```python
from build123d import *


with BuildPart() as part:
    # Sweep1: sweep along a path in Sketch1
    with BuildLine(Plane(origin=(0, 0, 0), x_dir=(1, 0, 0), z_dir=(0, 1, 0))) as sweep1_path:
        Line((0, 0), (25.4, 0))
        ThreePointArc((25.4, 0), (30.4, 1.339745962), (34.060254038, 5))
    # Sketch2 → Sweep1 (sweep)
    with BuildSketch(Plane(origin=(0, 0, 0), x_dir=(0, 0, -1), z_dir=(1, 0, 0))):
        with BuildLine():
            Line((0, 5), (0, -5))
            Line((0, -5), (-5, -5))
            ThreePointArc((-5, -5), (-3.974330816, 0), (-5, 5))
            Line((-5, 5), (0, 5))
        make_face()
    sweep(path=sweep1_path.line)


solid = part.part
```
The model under review builds one solid part; all positions refer to its coordinate system, in mm. A direction names the side the tool comes from. Round coordinates to 2 decimals unless told otherwise and drop trailing zeros. Loops run counter-clockwise (first coordinate to the right, second up) from the corner with the lowest first, then second, coordinate; pieces in that order, holes last.
1) Tool access review of faces 4 (the face through (13, 0, 0)), 5 (the face through (0, 0, 2)): name each direction out of +Z, -Z, +X, -X, +Y, -Y from which nothing blocks a thin tool from reaching the whole face with its end or side.
Values follow:
face 4: -Z, -X, +Y, -Y
face 5: +Z, -Z, -X, +Y, -Y
2) Wall thickness on line 1 along Z through (x, y) = (6.5, -3); line 2 along Z through (x, y) = (3, 0.25); line 3 along X through (y, z) = (4.75, -3.25): over which ranges is each line inside the solid? List them lowest first.
Values follow:
line 1: z = 0 to 4.33
line 2: z = 0 to 3.98
line 3: x = 32.78 to 37.09
3) The part is to be moulded in two halves that separate along X. For faces 1 (the face through (35.775, 0.07, -4.01)), 2 (the face through (30.336, 0.07, -1.303)), 3 (the face through (19, -5, 1)), say which applies: pulls with the +X half, pulls with the -X half, needs draft (parallel to the pull), parting line crosses it, or undercut.
Values follow:
face 1: pulls with the +X half
face 2: pulls with the -X half
face 3: needs draft
4) Consider section C-C on y = 3.25. State the section outline as (x, z) points, then the cut area to 3 significant figures.
Values follow:
outline: (0, 0) - (25.4, 0) arc R10 cw to (34.06, -5) - (37.87, -2.8) arc R14.4 ccw to (25.4, 4.4) - (0, 4.4) - close
area: 168 mm2
5) Consider section B-B on x = 24.5. State the section outline as (y, z) points, then the cut area to 3 significant figures.
Values follow:
outline: (-5, 0) - (5, 0) - (5, 5) arc R12.7 cw to (-5, 5) - close
area: 43.1 mm2
6) Consider section A-A on y = 1.75. State the section outline as (x, z) points.
Values follow:
outline: (0, 0) - (25.4, 0) arc R10 cw to (34.06, -5) - (37.61, -2.95) arc R14.1 ccw to (25.4, 4.1) - (0, 4.1) - close
7) Clearance check with flat-ended pins moving along their axes: P1, Ø3, axis at x = 18.5, y = -2.5, coming from the -Z side; P2, Ø2, axis at x = 24, y = 0.5, coming from the +Z side; P3, Ø1.5, axis at y = 0, z = 0, coming from the +X side. State where each tip first meets the part, or that it passes through.
Values follow:
P1: stops at z = 0
P2: stops at z = 4.06
P3: stops at x = 35.87
